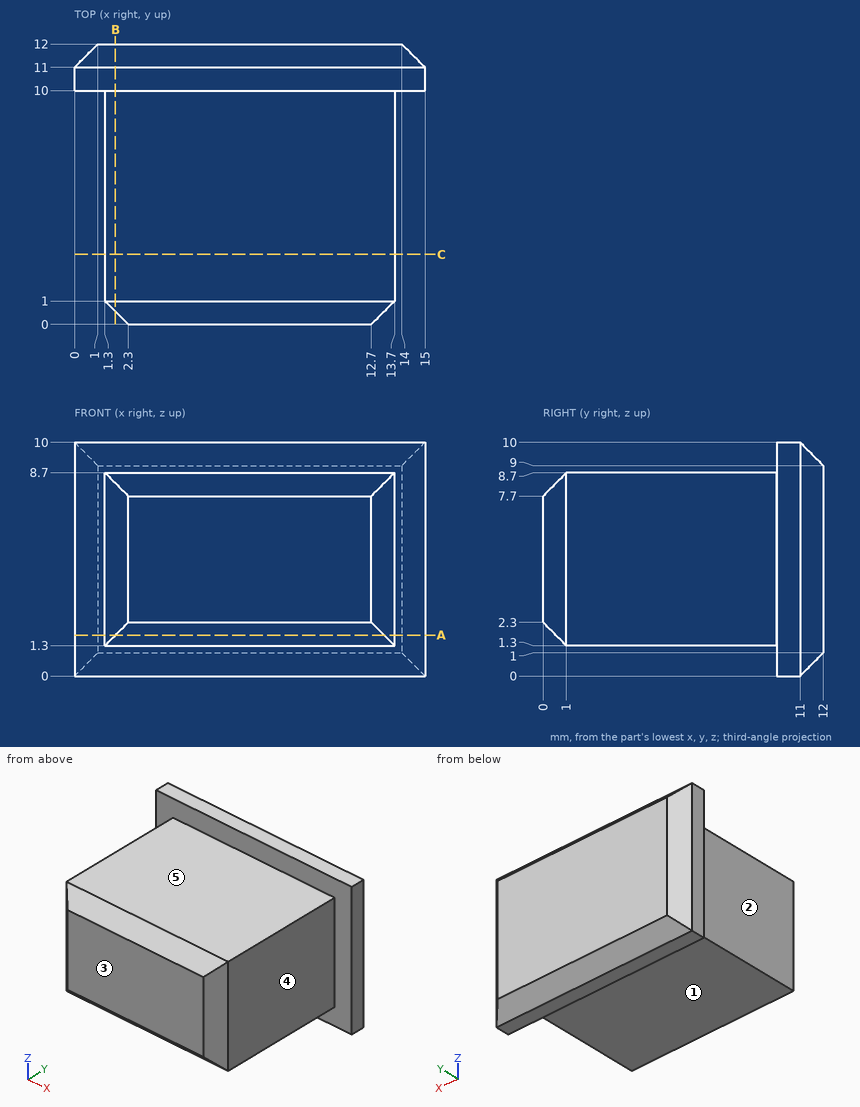
Drawing for the job (mm, zero at the part's lowest x, y, z). A direction names the side the tool comes from. Give positions to 0.01 mm unless a question says otherwise; leave off trailing zeros. Order: outer loops, then holes, each group sorted by start corner. A loop starts at its lowest first (then second) coordinate and runs counter-clockwise, first axis right, second up. Notation, with made-up numbers: M 23,-8.5 L 49,-8.5 A26 ccw 49,24.5 Z; hole C 42,9.25 d1. An arc over 180 degrees is marked long. Put each result on its own line as item: value. Start each with the question number.
(1) Which spindle directions (+Z, -Z, +X, -X, +Y, -Y) get a long thin tool onto all of the face, cutting with end or side? Do the marked faces 1, 2, 3, 4 and 5. Say none if no direction does.
(2) Saw through at C-C, the plane y = 3. Write the cut outline in (x, z).
(3) Drill centre lines: line 1 along X through (y, z) = (2.75, 3); line 2 along Z through (x, y) = (9.25, 8.5); line 3 along Y through (x, z) = (3, 1.25). Where is each one in solid material? Low to high.
(4) Flat gauge pins, fed straight in: pin 1 Ø1 at (x, y) = (7, 8) entering from -Z; pin 2 Ø4.5 at (x, y) = (10.5, 3.5) entering from +Z; pin 3 Ø1 at (y, z) = (2.5, 8) entering from -X. Where does each tip first touch, or does it go through?
(5) Saw through at B-B, the plane x = 1.75. Write the cut outline in (y, z), then the cut area to 3 significant figures.
(6) Saw through at A-A, the plane z = 1.75. Write the cut outline in (x, y), then the cut area to 3 significant figures.
Check result:
1. face 1: -Z, +X, -X, -Y
1. face 2: +Z, -Z, -X, -Y
1. face 3: +Z, -Z, +X, -X, -Y
1. face 4: +Z, -Z, +X, -Y
1. face 5: +Z, +X, -X, -Y
2. outline: M 1.3,1.3 L 13.7,1.3 L 13.7,8.7 L 1.3,8.7 Z
3. line 1: x = 1.3 to 13.7
3. line 2: z = 1.3 to 8.7
3. line 3: y = 10 to 12
4. pin 1: stops at z = 1.3
4. pin 2: stops at z = 8.7
4. pin 3: stops at x = 1.3
5. outline: M 0.55,1.75 L 1,1.3 L 10,1.3 L 10,0 L 11,0 L 12,1 L 12,9 L 11,10 L 10,10 L 10,8.7 L 1,8.7 L 0.55,8.25 Z
5. area: 88.7 mm2
6. outline: M 0,10 L 1.3,10 L 1.3,1 L 1.75,0.55 L 13.25,0.55 L 13.7,1 L 13.7,10 L 15,10 L 15,11 L 14,12 L 1,12 L 0,11 Z
6. area: 146 mm2
